Could you check a few things on this drawing? It's one solid part, dimensions in mm from its lowest x, y, z. A direction names the side the tool comes from. Give positions to 0.01 mm unless a question says otherwise; leave off trailing zeros. Write each loop counter-clockwise with the first axis right and the second up, starting at its lowest first coordinate (ties: lowest second). Pieces come first, ordered by that corner, then holes. Notation, with made-up numbers: (-4, 42) -> (17, 42) arc R27 cw to (17, 60) -> close; hole circle Ø5 at (37.25, 76.5). An arc over 180 degrees is marked (long way). Use CSV: the item, a comma, the result in double quotes. Start each with the question number.
(1) Suppose I cut it at B-B on z = 9.25. List the corners of the cut face in (x, y) for me.
(2) For pin 1 Ø1.5 at (y, z) = (4.5, 10) entering from -X; pin 2 Ø1.2 at (x, y) = (2.5, 2.5) entering from +Z; pin 3 Ø1.5 at (x, z) = (4, 5.5) entering from +Y (1 decimal), each with a flat end and sliding along its axis, tell me the tip position at first contact or that it passes through.
(3) Which directions (+Z, -Z, +X, -X, +Y, -Y) give clear straight access to the entire face, cutting with the end or side of a thin tool? Please do the marked faces 1 and 2.
(4) If we mould it in two halves opening along Y, with no side actions, what happens to the marked faces 3, 4 and 5? For each: pulls with the +Y half, pulls with the -Y half, needs draft (parallel to the pull), parting line crosses it, or undercut.
(5) I need wall thicknesses on L1, parallel to Z at x = 3.05, y = 2.1; L2, parallel to Z at x = 2.3, y = 0.9; L3, parallel to X at y = 3.7, z = 12 (1 decimal). Which ranges of each line are inside material? Lowest first, please. Write a range as [from, to].
(6) Suppose I cut it at A-A on y = 2.75. List the corners of the cut face in (x, z) for me.
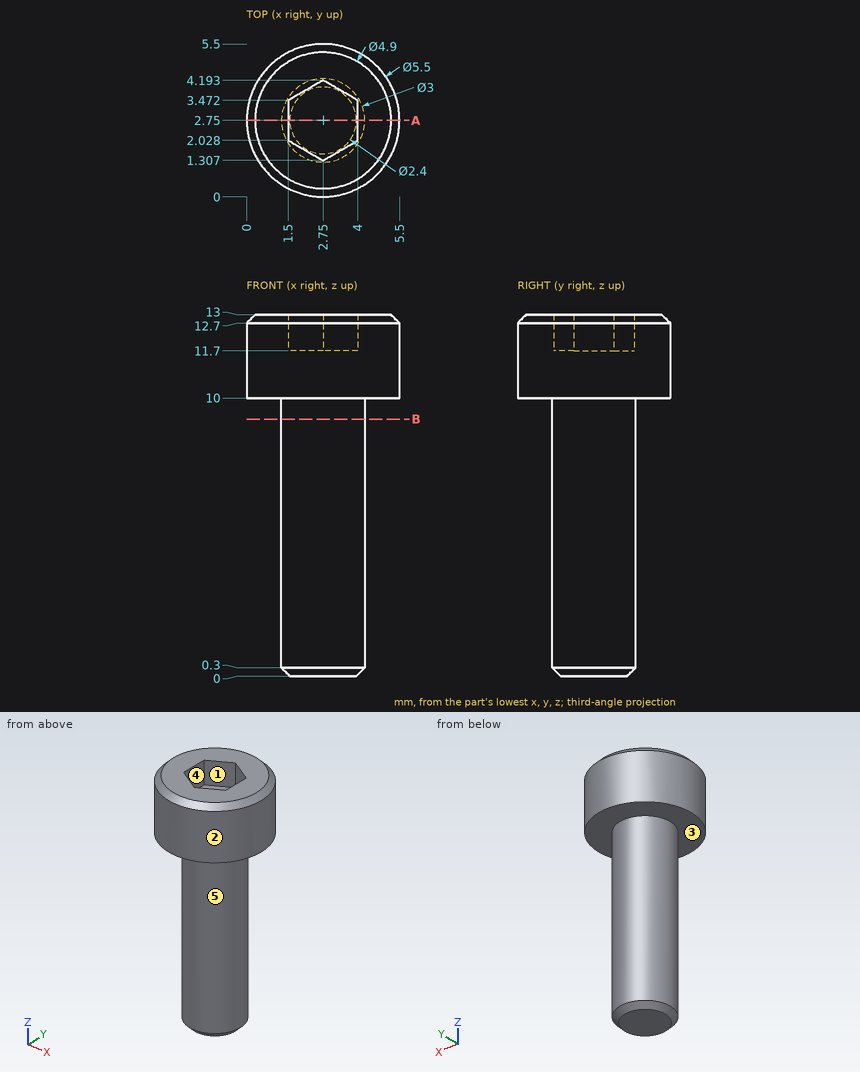
Geometry says:
1,outline,"circle Ø3 at (2.75, 2.75)"
2,pin 1,"x = 0.19"
2,pin 2,"z = 11.7"
2,pin 3,"y = 4.2"
3,face 1,"+Z"
3,face 2,"+Z, -Z"
4,face 3,"needs draft"
4,face 4,"undercut"
4,face 5,"parting line crosses it"
5,L1,"[0, 11.7]"
5,L2,"[10, 13]"
5,L3,"[0.2, 1.9], [3.6, 5.3]"
6,outline,"(0, 10) -> (1.25, 10) -> (1.25, 0.3) -> (1.55, 0) -> (3.95, 0) -> (4.25, 0.3) -> (4.25, 10) -> (5.5, 10) -> (5.5, 12.7) -> (5.2, 13) -> (4, 13) -> (4, 11.7) -> (1.5, 11.7) -> (1.5, 13) -> (0.3, 13) -> (0, 12.7) -> close"
